Geometry check sheet. Reference: the model listing, model coordinates, mm. Face numbers are marked on the shaded views. A direction names the side the tool comes from. Round coordinates to 2 decimals unless told otherwise and drop trailing zeros. Order: outer loops, then holes, each group sorted by start corner. A loop starts at its lowest first (then second) coordinate and runs counter-clockwise, first axis right, second up. Notation, with made-up numbers: M 53,11 L 100,11 A10 cw 100,25 Z; hole C 8.25,-16 d6. An arc over 180 degrees is marked long. Answer as a JSON object with one key per item and string values. Group by question number.
Autodesk Inventor part; units mm, degrees
ref_plane "YZ Plane" through (0, 0, 0) normal (1, 0, 0) x (0, 1, 0)
ref_plane "XZ Plane" through (0, 0, 0) normal (0, 1, 0) x (-1, 0, 0)
ref_plane "XY Plane" through (0, 0, 0) normal (0, 0, 1) x (1, 0, 0)
sketch "Sketch1" plane through (0, 0, 0) normal (0, 1, 0) x (-1, 0, 0)
  line L0 (0, 0) -> (4.4, 0)
  line L1 (4.4, 0) -> (4.4, -6.16)
  line L2 (4.4, -6.16) -> (0, -6.16)
  line L3 (0, -6.16) -> (0, 0)
  dimension "d0" = 6.16
  dimension "d1" = 4.4
extrude "Extrusion1" add sketch "Sketch1" along normal blind 4.6
sketch "Sketch2" plane through (0, 4.6, 0) normal (0, 1, 0) x (1, 0, 0)
  line L0 (-3.9333, 1.23) -> (-2.4333, 1.23)
  line L1 (-2.4333, 1.23) -> (-2.4333, 4.93)
  line L2 (-2.4333, 4.93) -> (-3.9333, 4.93)
  line L3 (-3.9333, 4.93) -> (-3.9333, 1.23)
  line L4 (-1.9667, 1.23) -> (-0.4667, 1.23)
  line L5 (-0.4667, 1.23) -> (-0.4667, 4.93)
  line L6 (-0.4667, 4.93) -> (-1.9667, 4.93)
  line L7 (-1.9667, 4.93) -> (-1.9667, 1.23)
  line L8 (-4.4, 0) -> (0, 0)
  line L9 (0, 0) -> (0, 6.16)
  line L10 (0, 6.16) -> (-4.4, 6.16)
  line L11 (-4.4, 6.16) -> (-4.4, 0)
  dimension "d4" = 3.7
  dimension "d5" = 1.5
  dimension "d6" = 4.4
  dimension "d7" = 0.4667
  dimension "d8" = 0.4667
  dimension "d9" = 6.16
  dimension "d10" = 1.23
extrude "Extrusion2" cut sketch "Sketch2" against normal blind 0.05 contours L3 L2 L1 L0 | L7 L6 L5 L4
sketch "Sketch4" plane through (0, 0, 0) normal (0, -1, 0) x (1, 0, 0)
  line L0 (-3.45, -1.58) -> (-3.05, -1.58)
  line L1 (-3.05, -1.58) -> (-3.05, -2.03)
  line L2 (-3.05, -2.03) -> (-3.45, -2.03)
  line L3 (-3.45, -2.03) -> (-3.45, -1.58)
  line L4 (-1.35, -1.58) -> (-0.95, -1.58)
  line L5 (-0.95, -1.58) -> (-0.95, -2.03)
  line L6 (-0.95, -2.03) -> (-1.35, -2.03)
  line L7 (-1.35, -2.03) -> (-1.35, -1.58)
  line L8 (-3.45, -4.13) -> (-3.05, -4.13)
  line L9 (-3.05, -4.13) -> (-3.05, -4.58)
  line L10 (-3.05, -4.58) -> (-3.45, -4.58)
  line L11 (-3.45, -4.58) -> (-3.45, -4.13)
  line L12 (-1.35, -4.13) -> (-0.95, -4.13)
  line L13 (-0.95, -4.13) -> (-0.95, -4.58)
  line L14 (-0.95, -4.58) -> (-1.35, -4.58)
  line L15 (-1.35, -4.58) -> (-1.35, -4.13)
  line L16 (0, 0) -> (-4.4, 0)
  line L17 (-4.4, 0) -> (-4.4, -6.16)
  line L18 (-4.4, -6.16) -> (0, -6.16)
  line L19 (0, -6.16) -> (0, 0)
  dimension "d13" = 0.45
  dimension "d14" = 0.4
  dimension "d15" = 2.5
  dimension "d16" = 3
  dimension "d17" = 4.4
  dimension "d18" = 6.16
  dimension "d19" = 1.58
  dimension "d20" = 0.95
extrude "Extrusion3" add sketch "Sketch4" along normal blind 24 contours L0 L1 L2 L3 | L4 L5 L6 L7 | L8 L9 L10 L11 | L12 L13 L14 L15
equation "\"d7\" = -0.666667 * d5 + 0.333333 * d6"
equation "\"d8\" = d7"
equation "\"d10\" = -0.5 * d4 + 0.5 * d9"
equation "\"d19\" = -0.5 * d16 + 0.5 * d18"
equation "\"d20\" = -0.5 * d15 + 0.5 * d17"
properties part number "LineSensor"
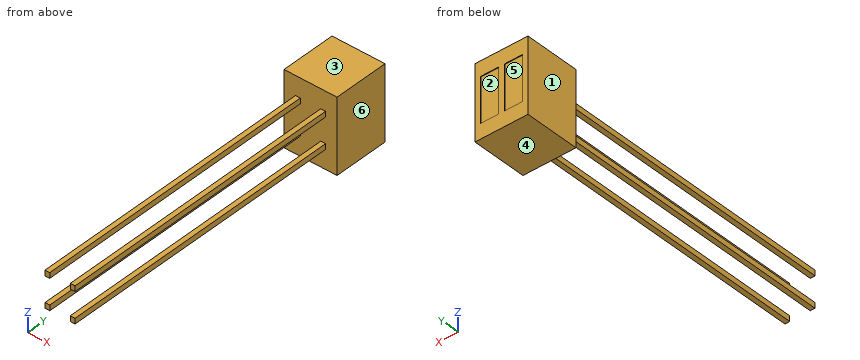
1) Sectioned sample at A-A (y = -9.5). Record the boundary of the cut face in (x, z), then the cut area to 3 significant figures.
2) Sectioned sample at B-B (z = -3.5). Record the boundary of the cut face in (x, y).
3) Release check for a two-part mould opening along Z. For the marked faces 3, 4, 5 and 6 record: +Z half, -Z half, draft (parallel to the pull), parting line (faces both ways), or undercut.
4) Set-up check for the marked faces 1 and 2: record each of +Z, -Z, +X, -X, +Y, -Y from which the full face is reachable in a straight line by a thin tool's end or side.
5) Sectioned sample at C-C (x = -2.8). Record the boundary of the cut face in (y, z).
6) Thickness scan on line 1 along Z through (x, y) = (-1.2, -20.25); line 2 along Y through (x, z) = (-1.4, -4). Record the ranges inside material, lowest first. Write a range as [from, to].
7) Go/stop test with flat-tipped pins: P1, Ø1, axis at y = -11.5, z = -4, coming from the +X side; P2, Ø2, axis at x = -2.5, y = -2.5, coming from the -Z side. Record where each tip stops, or that it passes through.
Final values:
{
 "1": {"outline": "M -3.45,-4.58 L -3.05,-4.58 L -3.05,-4.13 L -3.45,-4.13 Z; M -3.45,-2.03 L -3.05,-2.03 L -3.05,-1.58 L -3.45,-1.58 Z; M -1.35,-4.58 L -0.95,-4.58 L -0.95,-4.13 L -1.35,-4.13 Z; M -1.35,-2.03 L -0.95,-2.03 L -0.95,-1.58 L -1.35,-1.58 Z", "area": "0.720 mm^2"},
 "2": {"outline": "M -4.4,0 L 0,0 L 0,4.6 L -0.47,4.6 L -0.47,4.55 L -1.97,4.55 L -1.97,4.6 L -2.43,4.6 L -2.43,4.55 L -3.93,4.55 L -3.93,4.6 L -4.4,4.6 Z"},
 "3": {"face 3": "+Z half", "face 4": "-Z half", "face 5": "undercut", "face 6": "draft"},
 "4": {"face 1": "+Z, -Z, -X, +Y, -Y", "face 2": "+Y"},
 "5": {"outline": "M 0,-6.16 L 4.6,-6.16 L 4.6,-4.93 L 4.55,-4.93 L 4.55,-1.23 L 4.6,-1.23 L 4.6,0 L 0,0 Z"},
 "6": {"line 1": "z = [-4.58, -4.13], [-2.03, -1.58]", "line 2": "y = [0, 4.55]"},
 "7": {"P1": "stops at x = -0.95", "P2": "stops at z = -4.58"}
}
